Work out the finished part from the listing and answer in its coordinate system (mm). Coordinates: 2 decimals unless noted, no trailing zeros. Loops run counter-clockwise (first coordinate to the right, second up) from the corner with the lowest first, then second, coordinate; pieces in that order, holes last. Notation, with made-up numbers: (20.25, -39.75) - (25.25, -39.75) arc R21 cw to (25.25, -17.75) - close; hole circle Ø1 at (12.25, 14). An arc over 180 degrees is marked (long way). Write each question's results on one line, items separated by ' | '. Start each with the question number.
1. Determine the mould class of faces 1 (the cylindrical face through (-0.59, 4.46, -0.06)), 2 (the flat face through (0, -5, -4.5)), 3 (the conical face through (3.288, 6.321, -4.375)), 4 (the flat face through (-3.95, -6.72, 0.05)) for opening direction Y: released by +Y, released by -Y, zero draft, split by the parting line, or undercut.
2. A cutting plane is placed at A-A on z = -4. Determine the outline of the cut face in (x, y).
3. Find the intervals of material crossed by line 1 along Y through (x, z) = (0.5, -1); line 2 along Y through (x, z) = (1, 1); line 3 along X through (y, z) = (3.5, 0.5), in increasing order. Write a range as [from, to].
4. This flat-tipped pin is pushed along its axis until it touches: P1, Ø3, axis at x = 5, z = 0, coming from the +Y side. Where does it stop, or does it pass through?
5. A cutting plane is placed at B-B on z = -2.75. Determine the outline of the cut face in (x, y), then the cut area to 3 significant figures.
from build123d import *

# Parameters (mm, degrees)
SKETCH1_R           = 4.5
BOSS_EXTRUDE1_DEPTH = 4.5
SKETCH2_OUTSIDE_W   = 40.68
SKETCH2_OUTSIDE_H   = 43.092
SKETCH2_OUTSIDE_R   = 7
CUT_EXTRUDE1_DEPTH  = 9
CUT_EXTRUDE1_TAPER  = 45


with BuildPart() as part:
    # Sketch1 → Boss-Extrude1 (new body, symmetric)
    with BuildSketch(Plane.XY):
        Polygon((7.794228634, -4.5), (7.794228634, 4.5), (0, 9), (-7.794228634, 4.5), (-7.794228634, -4.5), (0, -9), align=None)
        Circle(SKETCH1_R, mode=Mode.SUBTRACT)
    extrude(amount=BOSS_EXTRUDE1_DEPTH, both=True)

    # Sketch2 outside → Cut-Extrude1 (cut)
    with BuildSketch(Plane.XY.offset(4.5)):
        Rectangle(SKETCH2_OUTSIDE_W, SKETCH2_OUTSIDE_H)
        Circle(SKETCH2_OUTSIDE_R, mode=Mode.SUBTRACT)
    cut_extrude1 = extrude(amount=-CUT_EXTRUDE1_DEPTH, taper=CUT_EXTRUDE1_TAPER, mode=Mode.SUBTRACT)

    # Mirror1: Cut-Extrude1 across plane
    add(cut_extrude1.mirror(Plane.XY), mode=Mode.SUBTRACT)


solid = part.part
Values:
1) face 1: undercut | face 2: zero draft | face 3: split by the parting line | face 4: released by -Y
2) outline: circle Ø15 at (0, 0); hole circle Ø9 at (0, 0)
3) line 1: [-8.71, -4.47], [4.47, 8.71] | line 2: [-8.42, -4.39], [4.39, 8.42] | line 3: [-7.79, -2.83], [2.83, 7.79]
4) P1: y = 6.98
5) outline: (-7.79, -3.98) arc R8.75 ccw to (-7.34, -4.76) - (-0.45, -8.74) arc R8.75 ccw to (0.45, -8.74) - (7.34, -4.76) arc R8.75 ccw to (7.79, -3.98) - (7.79, 3.98) arc R8.75 ccw to (7.34, 4.76) - (0.45, 8.74) arc R8.75 ccw to (-0.45, 8.74) - (-7.34, 4.76) arc R8.75 ccw to (-7.79, 3.98) - close; hole circle Ø9 at (0, 0) | area: 146 mm^2
